Geometry: final body of the model. Coordinates: model frame, mm. A direction names the side the tool comes from. Give positions to 0.01 mm unless a question says otherwise; leave off trailing zeros. Write each loop counter-clockwise with the first axis right and the second up, starting at its lowest first coordinate (ties: lowest second). Pieces come first, ordered by that corner, then holes.
from build123d import *

# Parameters (mm, degrees)
SKETCH_1_W          = 432
SKETCH_1_H          = 522
SKETCH_1_W_2        = 430
SKETCH_1_H_2        = 520
EXTRUDE_2_DEPTH     = 330
SKETCH_2_W          = 82
SKETCH_2_H          = 220
CUT_EXTRUDE_2_DEPTH = 10
SKETCH_3_W          = 200
SKETCH_3_H          = 150
CUT_EXTRUDE_3_DEPTH = 10


with BuildPart() as part:
    # Эскиз1 → Вытянуть-Тонкостенный2 (new body)
    with BuildSketch(Plane(origin=(0, 0, 0), x_dir=(1, 0, 0), z_dir=(0, 1, 0))):
        with Locations((-215, 260)):
            Rectangle(SKETCH_1_W, SKETCH_1_H)
        with Locations((-215, 260)):
            Rectangle(SKETCH_1_W_2, SKETCH_1_H_2, mode=Mode.SUBTRACT)
    extrude(amount=EXTRUDE_2_DEPTH)

    # Эскиз2 → Вырез-Вытянуть2 (cut)
    with BuildSketch(Plane(origin=(1, 0, 0), x_dir=(0, 0, -1), z_dir=(1, 0, 0))):
        with Locations((83, 120)):
            Rectangle(SKETCH_2_W, SKETCH_2_H)
    extrude(amount=-CUT_EXTRUDE_2_DEPTH, mode=Mode.SUBTRACT)

    # Эскиз3 → Вырез-Вытянуть3 (cut)
    with BuildSketch(Plane(origin=(0, 0, -521), x_dir=(-1, 0, 0), z_dir=(0, 0, -1))):
        with Locations((189, 155)):
            Rectangle(SKETCH_3_W, SKETCH_3_H)
    extrude(amount=-CUT_EXTRUDE_3_DEPTH, mode=Mode.SUBTRACT)


solid = part.part
Q1. Pin query (flat end, axial travel): P1, Ø1.1, axis at x = -139.5, z = -520.5, coming from the -Y side; P2, Ø4, axis at y = 105.5, z = -56.5, coming from the +X side. Return the tip coordinate at first contact, or that it passes through.
Filled sheet:
P1: stops at y = 0
P2: stops at x = -430
Q2. Pull-direction query (Z, two-part tool) for faces 3 (the flat face through (-218, 236, -521)), 4 (the flat face through (-218, 163, 0)), 5 (the flat face through (1, 163, -256)), 6 (the flat face through (-218, 163, 1)); classes: released by +Z, released by -Z, zero draft, split by the parting line, or undercut.
Filled sheet:
face 3: released by -Z
face 4: undercut
face 5: zero draft
face 6: released by +Z
Q3. Access query for faces 1 (the flat face through (-431, 163, -256)), 2 (the flat face through (-430, 163, -256)). Directions: +Z, -Z, +X, -X, +Y, -Y. A direction counts if a zero-diameter tool reaches every point of the face in a straight line with its end or side. Return the directions, or none.
Filled sheet:
face 1: +Z, -Z, -X, +Y, -Y
face 2: +Y, -Y
Q4. Ray query, line 1 along X through (y, z) = (265, -27.5); line 2 along Z through (x, y) = (-142, 70.5); line 3 along Z through (x, y) = (-245, 110.5). Return the intervals inside material, ascending.
Filled sheet:
line 1: x = -431 to -430, 0 to 1
line 2: z = -521 to -520, 0 to 1
line 3: z = 0 to 1
Q5. Section C-C on y = 151. Output: boundary loops of the cut face in (x, z), plus the area to 3 significant figures.
Filled sheet:
outline: (-431, -521) - (-289, -521) - (-289, -520) - (-430, -520) - (-430, 0) - (0, 0) - (0, -42) - (1, -42) - (1, 1) - (-431, 1) - close; (-89, -521) - (1, -521) - (1, -124) - (0, -124) - (0, -520) - (-89, -520) - close
area: 1,620 mm2
Q6. Section A-A on x = -264. Output: boundary loops of the cut face in (y, z).
Filled sheet:
outline: (0, -521) - (80, -521) - (80, -520) - (0, -520) - close; (0, 0) - (330, 0) - (330, 1) - (0, 1) - close; (230, -521) - (330, -521) - (330, -520) - (230, -520) - close
Q7. Section B-B on x = -339.5. Output: boundary loops of the cut face in (y, z), plus the area to 3 significant figures.
Filled sheet:
outline: (0, -521) - (330, -521) - (330, -520) - (0, -520) - close; (0, 0) - (330, 0) - (330, 1) - (0, 1) - close
area: 660 mm2
Q8. Section D-D on z = -324. Output: boundary loops of the cut face in (x, y).
Filled sheet:
outline: (-431, 0) - (-430, 0) - (-430, 330) - (-431, 330) - close; (0, 0) - (1, 0) - (1, 330) - (0, 330) - close
